Here's how the part is built. I have some questions about the finished solid (model axes, mm). Coordinates: 2 decimals unless noted, no trailing zeros. Write each loop counter-clockwise with the first axis right and the second up, starting at its lowest first coordinate (ties: lowest second). Pieces come first, ordered by that corner, then holes.
Item 1: If we section it at C-C (x = 19.5): Count the separate pieces of the cut face and the enclosed holes in it, then the cut area to 3 significant figures.
Item 2: If we section it at A-A (x = 0): Please give me the cut outline in (y, z), then the cut area to 3 significant figures.
Item 3: I'm going to push flat-ended pins straight in: pin 1 Ø22.5 at (x, y) = (-18.02, -10.4) entering from +Z; pin 2 Ø1 at (y, z) = (-22, 4.5) entering from -X; pin 3 Ø6 at (x, z) = (5.5, 4) entering from +Y; pin 4 Ø4 at (x, y) = (-31.5, -28.5) entering from -Z. Where does each tip first touch, or does it pass through?
Item 4: If we section it at B-B (z = -3.75): Please give me the cut outline in (x, y) (1 decimal).
Item 5: If I drill on line 1 (Y direction, x = -21, z = -1); line 2 (Y direction, x = 23, z = -6); line 3 (Y direction, x = -6, z = 6), over which ranges is the centre line in solid material (lowest first)?
Item 6: We'd pull the mould along Z, two halves only. Please class faces 1 (the face through (35.47, -11.17, 0.89)), 2 (the face through (1, 8, -7.5)), 3 (the face through (-1, 8, 7.5)): +Z half, -Z half, draft (parallel to the pull), parting line (faces both ways), or undercut.
from build123d import *

# Parameters (mm, degrees)
F2_R          = 1
F3_R          = 7.62
F3_R_2        = 9.8425
F4_DEPTH      = 7.501
F4_DEPTH_BACK = 7.501


with BuildPart() as f1:
    # F0 (on Front) → F1 (revolve)
    with BuildSketch(Plane.XZ):
        with BuildLine():
            Line((41.5925, 7.5), (0, 7.5))
            Line((0, 7.5), (0, -7.5))
            Line((0, -7.5), (41.5925, -7.5))
            Line((41.5925, -7.5), (36.9623001308, -0.5547001962))
            ThreePointArc((36.9623001308, -0.5547001962), (36.7943504252, 0), (36.9623001308, 0.5547001962))
            Line((36.9623001308, 0.5547001962), (41.5925, 7.5))
        make_face()
    revolve(axis=Axis((0, 0, 0), (0, 0, -1)))

    # F2
    f2_edges = [f1.edges().sort_by_distance(p)[0] for p in [
        (-41.5925, 0, 7.5),
        (-41.5925, 0, -7.5),
    ]]
    fillet(f2_edges, radius=F2_R)

    # F3 (on Top) → F4 (cut, two sides)
    with BuildSketch(Plane.XY) as f4_sk:
        Circle(F3_R)
        with Locations((0, 20.8075332025)):
            Circle(F3_R_2)
        with Locations((-18.0198523435, 10.4037666013)):
            Circle(F3_R_2)
        with Locations((-18.0198523435, -10.4037666013)):
            Circle(F3_R_2)
        with Locations((0, -20.8075332025)):
            Circle(F3_R_2)
        with Locations((18.0198523435, -10.4037666013)):
            Circle(F3_R_2)
        with Locations((18.0198523435, 10.4037666013)):
            Circle(F3_R_2)
    extrude(amount=-F4_DEPTH, mode=Mode.SUBTRACT)
    extrude(f4_sk.sketch, amount=F4_DEPTH_BACK, mode=Mode.SUBTRACT)


solid = f1.part
Answer list:
1. separate pieces: 3
1. enclosed holes: 0
1. area: 429 mm2
2. outline: (-40.56, -5.95) arc R1 ccw to (-39.72, -7.5) - (-30.65, -7.5) - (-30.65, 7.5) - (-39.72, 7.5) arc R1 ccw to (-40.56, 5.95) - (-36.96, 0.55) arc R1 cw to (-36.96, -0.55) - close; (-10.97, -7.5) - (-7.62, -7.5) - (-7.62, 7.5) - (-10.97, 7.5) - close; (7.62, -7.5) - (10.97, -7.5) - (10.97, 7.5) - (7.62, 7.5) - close; (30.65, -7.5) - (39.72, -7.5) arc R1 ccw to (40.56, -5.95) - (36.96, -0.55) arc R1 cw to (36.96, 0.55) - (40.56, 5.95) arc R1 ccw to (39.72, 7.5) - (30.65, 7.5) - close
2. area: 351 mm2
3. pin 1: stops at z = 7.5
3. pin 2: stops at x = -33.43
3. pin 3: stops at y = 40.55
3. pin 4: stops at z = -7.16
4. outline: circle Ø78.2 at (0, 0); hole circle Ø19.7 at (-18, -10.4); hole circle Ø19.7 at (-18, 10.4); hole circle Ø19.7 at (0, -20.8); hole circle Ø19.7 at (0, 20.8); hole circle Ø15.2 at (0, 0); hole circle Ø19.7 at (18, -10.4); hole circle Ø19.7 at (18, 10.4)
5. line 1: y = -30.78 to -19.78, -1.02 to 1.02, 19.78 to 30.78
5. line 2: y = -33.44 to -18.89, -1.91 to 1.91, 18.89 to 33.44
5. line 3: y = -40.14 to -28.61, -13.01 to -4.7, 4.7 to 13.01, 28.61 to 40.14
6. face 1: undercut
6. face 2: -Z half
6. face 3: +Z half
